from build123d import *

# Parameters (mm, degrees)
F0_W          = 45.31
F0_H          = 30
F0_R          = 8
F1_DEPTH      = 15
F2_W          = 1.1
F2_H          = 12
F3_DEPTH      = 25
F3_DEPTH_BACK = 25
F5_W          = 59.0507443994
F5_H          = 44.4323215634
F5_R          = 10.3976804266
F5_R_2        = 11
F6_DEPTH      = 5
F7_R          = 10


with BuildPart() as f1:
    # F0 (on Front) → F1 (new body)
    with BuildSketch(Plane.XZ):
        with Locations((0, -1.6586469859)):
            Rectangle(F0_W, F0_H)
        with Locations((-13.03, 0)):
            Circle(F0_R, mode=Mode.SUBTRACT)
        with Locations((13.03, 0)):
            Circle(F0_R, mode=Mode.SUBTRACT)
    extrude(amount=F1_DEPTH)

    # F2 (on Right) → F3 (cut, two sides)
    with BuildSketch(Plane.YZ) as f3_sk:
        with Locations((-5.55, -13)):
            Rectangle(F2_W, F2_H)
    extrude(amount=-F3_DEPTH, mode=Mode.SUBTRACT)
    extrude(f3_sk.sketch, amount=F3_DEPTH_BACK, mode=Mode.SUBTRACT)

    # F5 (on offset) → F6 (cut)
    with BuildSketch(Plane.XZ.offset(15)):
        with Locations((2.6295455173, 0.7389681414)):
            Rectangle(F5_W, F5_H)
        with Locations((-13, 0)):
            Circle(F5_R, mode=Mode.SUBTRACT)
        with Locations((13, 0)):
            Circle(F5_R_2, mode=Mode.SUBTRACT)
    extrude(amount=-F6_DEPTH, mode=Mode.SUBTRACT)

    # F7
    f7_edges = [f1.edges().sort_by_distance(p)[0] for p in [
        (22.655, -5, 13.341353),
        (-22.655, -5, 13.341353),
    ]]
    fillet(f7_edges, radius=F7_R)


solid = f1.part
CAD build for the part. Positions are in the model's coordinates, mm. A direction names the side the tool comes from. Give positions to 0.01 mm unless a question says otherwise; leave off trailing zeros. Order: outer loops, then holes, each group sorted by start corner. A loop starts at its lowest first (then second) coordinate and runs counter-clockwise, first axis right, second up. Notation, with made-up numbers: (25, 8.25) -> (59, 8.25) arc R19 ccw to (59, 39.25) -> close; hole circle Ø3 at (46.25, 55.25). An arc over 180 degrees is marked (long way). Return JSON: item names as keys, results as strings.
Q1. Saw through at D-D (y = -10.5). Write the cut outline in (x, z) (3 decimals), then the cut area to 3 significant figures.
Working result:
{"outline": "(-22.655, -3.859) arc R10.398 ccw (long way) to (-22.64, 3.898) arc R10 ccw to (-22.655, 3.341) -> close; (22.349, 5.796) arc R11 ccw (long way) to (22.655, -5.271) -> (22.655, 3.341) arc R10 ccw to start; hole circle Ø16 at (-13.03, 0); hole circle Ø16 at (13.03, 0)", "area": "304 mm²"}
Q2. Flat gauge pins, fed straight in: pin 1 (1.5 mm diameter, centred on x = -12.5, z = -6, fed in from -Y); pin 2 (1 mm diameter, centred on x = -1.5, z = -1.5, fed in from -Y); pin 3 (0.9 mm diameter, centred on x = -4, y = -5.5, fed in from -Z). Where does each tip first touch, or does it go through?
Working result:
{"pin 1": "through", "pin 2": "y = -10", "pin 3": "z = -7"}
Q3. Drill centre lines: line 1 (Y direction, x = 2, z = -9); line 2 (Z direction, x = -13.03, y = -7.5); line 3 (X direction, y = -3.75, z = 5) (3 decimals). Where is each one in solid material? Low to high.
Working result:
{"line 1": "-10 to -6.1, -5 to 0", "line 2": "-16.66 to -8, 8 to 13.33", "line 3": "-22.516 to -19.275, -6.785 to 6.785, 19.275 to 22.516"}
Q4. Mould opens along Y. For faces 4 (the face through (0, 0, -1)), 5 (the face through (0, -5, -12)), 6 (the face through (-10, -15, -8)), 7 (the face through (22.655, -6, -5)) say: pulls with the +Y half, pulls with the -Y half, needs draft (parallel to the pull), parting line crosses it, or undercut.
Working result:
{"face 4": "pulls with the +Y half", "face 5": "undercut", "face 6": "pulls with the -Y half", "face 7": "needs draft"}
Q5. Saw through at C-C (z = -8.5). Write the cut outline in (x, y) (3 decimals).
Working result:
{"outline": "(-22.655, -10) -> (-18.988, -10) -> (-18.988, -15) -> (-7.012, -15) -> (-7.012, -10) -> (6.018, -10) -> (6.018, -15) -> (19.982, -15) -> (19.982, -10) -> (22.655, -10) -> (22.655, -6.1) -> (-22.655, -6.1) -> close; (-22.655, -5) -> (22.655, -5) -> (22.655, 0) -> (-22.655, 0) -> close"}
Q6. Which spindle directions (+Z, -Z, +X, -X, +Y, -Y) get a long thin tool onto all of the face, cutting with end or side? Do faces 1 (the face through (11.989, -7.395, 7.932)), 2 (the face through (-2.61, -12.54, -0.42)), 3 (the face through (-19.7, -5.6, -7)). Say none if no direction does.
Working result:
{"face 1": "+Y, -Y", "face 2": "-Y", "face 3": "-Z, +X, -X"}
Q7. Saw through at A-A (z = 0). Write the cut outline in (x, y) (3 decimals), then the cut area to 3 significant figures.
Working result:
{"outline": "(-22.655, -15) -> (-21.03, -15) -> (-21.03, 0) -> (-22.655, 0) -> close; (-5.03, -15) -> (-2.602, -15) -> (-2.602, -10) -> (2, -10) -> (2, -15) -> (5.03, -15) -> (5.03, 0) -> (-5.03, 0) -> close; (21.03, -15) -> (22.655, -15) -> (22.655, 0) -> (21.03, 0) -> close", "area": "177 mm²"}
Q8. Saw through at B-B (y = -3.5). Write the cut outline in (x, z) (3 decimals), then the cut area to 3 significant figures.
Working result:
{"outline": "(-22.655, -16.659) -> (22.655, -16.659) -> (22.655, 3.341) arc R10 ccw to (12.655, 13.341) -> (-12.655, 13.341) arc R10 ccw to (-22.655, 3.341) -> close; hole circle Ø16 at (-13.03, 0); hole circle Ø16 at (13.03, 0)", "area": "914 mm²"}
